Design review of the part built by this model. Coordinates are the model's own, in mm. Give positions to 0.01 mm unless a question says otherwise; leave off trailing zeros. Write each loop counter-clockwise with the first axis right and the second up, starting at its lowest first coordinate (ties: lowest second). Pieces come first, ordered by that corner, then holes. Notation, with made-up numbers: M 85,38 L 137,38 A20 cw 137,42 Z; hole C -25.75,-5.75 d11. An arc over 180 degrees is marked long. Answer in a Markdown table with one row per item.
```python
from build123d import *

# Parameters (mm, degrees)
F0_W     = 40
F0_H     = 80
F0_R     = 7.5
F1_DEPTH = 25


with BuildPart() as f1:
    # F0 (on Front) → F1 (new body)
    with BuildSketch(Plane.XZ):
        Rectangle(F0_W, F0_H)
        with Locations((0, 23.313124)):
            Circle(F0_R, mode=Mode.SUBTRACT)
        Polygon((-20, 40), (20, 40), (0, 74.641016), align=None)
    extrude(amount=F1_DEPTH)


solid = f1.part
```
1) Add section C-C (y = -15.75). Write out the cut boundary in (x, z).
Geometry says:
| item | result |
|---|---|
| outline | M -20,-40 L 20,-40 L 20,40 L 0,74.64 L -20,40 Z; hole C 0,23.31 d15 |
2) Add section B-B (x = -6). Write out the cut boundary in (y, z), and give its area (3 significant figures).
Geometry says:
| item | result |
|---|---|
| outline | M -25,-40 L 0,-40 L 0,18.81 L -25,18.81 Z; M -25,27.81 L 0,27.81 L 0,64.25 L -25,64.25 Z |
| area | 2,380 mm^2 |
3) Add section D-D (x = 16). Write out the cut boundary in (y, z), and give its area (3 significant figures).
Geometry says:
| item | result |
|---|---|
| outline | M -25,-40 L 0,-40 L 0,46.93 L -25,46.93 Z |
| area | 2,170 mm^2 |
4) To check wall thickness, follow probe 1 along Z at (x, y) = (1, -7.75); probe 2 along Z at (x, y) = (4, -4); probe 3 along Z at (x, y) = (13.5, -4.5). State the ranges of each line that lie inside material, in increasing order. Write a range as [from, to].
Geometry says:
| item | result |
|---|---|
| probe 1 | [-40, 15.88], [30.75, 72.91] |
| probe 2 | [-40, 16.97], [29.66, 67.71] |
| probe 3 | [-40, 51.26] |
5) The part is to be moulded in two halves that separate along Z. For faces 1 (the face through (0, -12, -40)), 2 (the face through (-0.98, -12.32, 30.75)), 3 (the face through (10.14, -12.32, 57.08)), 4 (the face through (0, 0, 5)), say which applies: released by +Z, released by -Z, zero draft, split by the parting line, or undercut.
Geometry says:
| item | result |
|---|---|
| face 1 | released by -Z |
| face 2 | undercut |
| face 3 | released by +Z |
| face 4 | zero draft |
6) Add section A-A (z = 29). Write out the cut boundary in (x, y).
Geometry says:
| item | result |
|---|---|
| outline | M -20,-25 L -4.89,-25 L -4.89,0 L -20,0 Z; M 4.89,-25 L 20,-25 L 20,0 L 4.89,0 Z |
7) Insertion check: P1, Ø1.5, axis at y = -13.5, z = 52, coming from the +X side; P2, Ø1.5, axis at x = -8, y = -7, coming from the +Z side. Each pin has a flat end and moves straight along its axis. Give the tip position at first contact, or say it passes through.
Geometry says:
| item | result |
|---|---|
| P1 | x = 13.5 |
| P2 | z = 62.08 |
